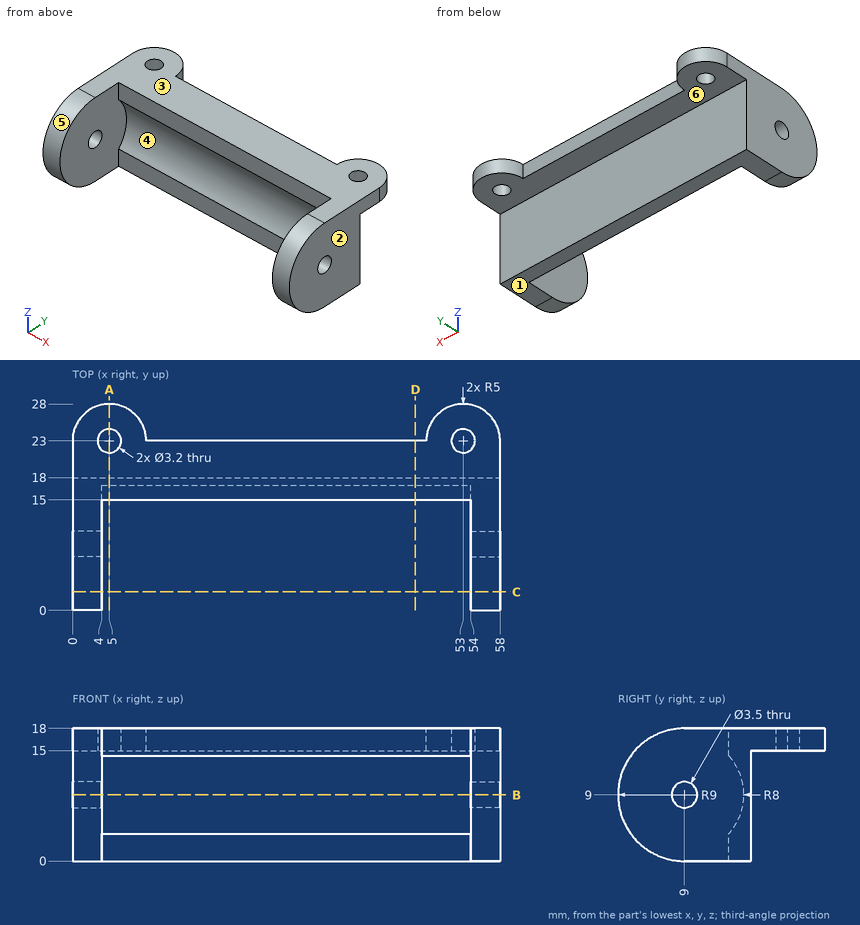
Part print with two shaded views. Sizes in mm from the minimum x, y, z corner. A direction names the side the tool comes from. Round coordinates to 2 decimals unless told otherwise and drop trailing zeros. Order: outer loops, then holes, each group sorted by start corner. A loop starts at its lowest first (then second) coordinate and runs counter-clockwise, first axis right, second up. Notation, with made-up numbers: (-6, 65) - (47, 65) arc R18 ccw to (47, 72) - close; hole circle Ø6 at (65.5, 47.5). An arc over 180 degrees is marked (long way). Answer in a Markdown table with one row per item. Add a question column.
(1) Band-saw the part on A-A on x = 5. List the corners of the cut face in (y, z), and give its area (3 significant figures).
(2) Mould opens along Z. For the marked faces 1, 2, 3 and 4 say: +Z half, -Z half, draft (parallel to the pull), parting line (faces both ways), or undercut.
(3) Drop flat-ended pins along their axis: pin 1 Ø1.9 at (x, z) = (30.5, 16.5) entering from -Y; pin 2 Ø1.5 at (x, z) = (36.5, 17) entering from +Y; pin 3 Ø3.5 at (x, y) = (5, 23) entering from -Z. Give the stop position or say it passes through.
(4) Band-saw the part on B-B on z = 9. List the corners of the cut face in (x, y), and give its area (3 significant figures).
(5) Band-saw the part on C-C on y = 2.5. List the corners of the cut face in (x, z).
(6) 3-axis set-ups, long thin cutter, end or side, ignore diameter. For the marked faces 5 and 6: which of +Z, -Z, +X, -X, +Y, -Y reach the whole face in a straight line?
(7) Probe L1, parallel to X at y = 8.5, z = 2; L2, parallel to Y at x = 1.3, z = 9; L3, parallel to Y at x = 53, z = 16.1. List the from-to ranges inside material, lowest first. Write a range as [from, to].
(8) Band-saw the part on D-D on x = 46.5. List the corners of the cut face in (y, z).
Data:
| question | item | result |
|---|---|---|
| 1 | outline | (15, 0) - (18, 0) - (18, 15) - (21.4, 15) - (21.4, 18) - (15, 18) - (15, 14.29) arc R8 cw to (15, 3.71) - close; (24.6, 15) - (28, 15) - (28, 18) - (24.6, 18) - close |
| 1 | area | 59.9 mm^2 |
| 2 | face 1 | -Z half |
| 2 | face 2 | draft |
| 2 | face 3 | +Z half |
| 2 | face 4 | undercut |
| 3 | pin 1 | stops at y = 15 |
| 3 | pin 2 | stops at y = 23 |
| 3 | pin 3 | stops at z = 15 |
| 4 | outline | (0, 0) - (4, 0) - (4, 7.25) - (0, 7.25) - close; (0, 10.75) - (4, 10.75) - (4, 17) - (54, 17) - (54, 10.75) - (58, 10.75) - (58, 18) - (0, 18) - close; (54, 0) - (58, 0) - (58, 7.25) - (54, 7.25) - close |
| 4 | area | 166 mm^2 |
| 5 | outline | (0, 2.78) - (4, 2.78) - (4, 15.22) - (0, 15.22) - close; (54, 2.78) - (58, 2.78) - (58, 15.22) - (54, 15.22) - close |
| 6 | face 5 | +X, -X, -Y |
| 6 | face 6 | -Z, +X, -X, +Y |
| 7 | L1 | x = [0, 4], [54, 58] |
| 7 | L2 | y = [0, 7.25], [10.75, 18] |
| 7 | L3 | y = [15, 21.4], [24.6, 28] |
| 8 | outline | (15, 0) - (18, 0) - (18, 15) - (23, 15) - (23, 18) - (15, 18) - (15, 14.29) arc R8 cw to (15, 3.71) - close |
